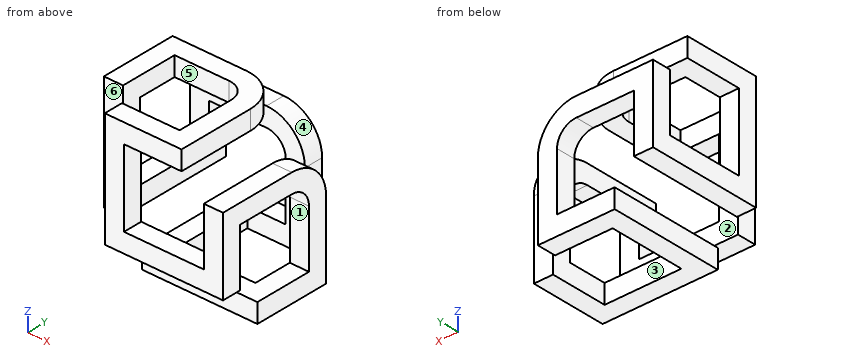
```python
from build123d import *

# Parameters (mm, degrees)
SKETCH_1_W      = 10
SKETCH_1_H      = 10
EXTRUDE_1_DEPTH = 10
EXTRUDE_2_DEPTH = 10
EXTRUDE_3_DEPTH = 10
EXTRUDE_4_DEPTH = 10
EXTRUDE_5_DEPTH = 10
EXTRUDE_6_DEPTH = 10
FILLET_3_R      = 20
FILLET_4_R      = 10
FILLET_5_R      = 20
FILLET_6_R      = 20
FILLET_7_R      = 10
FILLET_8_R      = 10


with BuildPart() as part:
    # 草图1 → 凸台-拉伸1 (new body)
    with BuildSketch(Plane.XY):
        Polygon((0, 60), (0, 30), (10, 30), (10, 50), (48.396471527, 50), (48.396471527, 10), (28.396471527, 10), (28.396471527, 0), (58.396471527, 0), (58.396471527, 60), align=None)
        with Locations((5, 25)):
            Rectangle(SKETCH_1_W, SKETCH_1_H)
        with Locations((23.396471527, 5)):
            Rectangle(SKETCH_1_W, SKETCH_1_H)
    extrude(amount=-EXTRUDE_1_DEPTH)

    # 草图2 → 凸台-拉伸2 (add)
    with BuildSketch(Plane.ZY):
        Polygon((0, 20), (-60, 20), (-60, 80), (-20, 80), (-20, 70), (-50, 70), (-50, 30), (-10, 30), (-10, 60), (0, 60), align=None)
    extrude(amount=-EXTRUDE_2_DEPTH)

    # 草图3 → 凸台-拉伸3 (add)
    with BuildSketch(Plane(origin=(0, 80, 0), x_dir=(1, 0, 0), z_dir=(0, 1, 0))):
        Polygon((0, 60), (0, 20), (60, 20), (60, 80), (20, 80), (20, 70), (50, 70), (50, 30), (10, 30), (10, 60), align=None)
    extrude(amount=-EXTRUDE_3_DEPTH)

    # 草图4 → 凸台-拉伸4 (add)
    with BuildSketch(Plane(origin=(0, 0, -80), x_dir=(-1, 0, 0), z_dir=(0, 0, -1))):
        Polygon((-60, 80), (-20, 80), (-20, 20), (-80, 20), (-80, 60), (-70, 60), (-70, 30), (-30, 30), (-30, 70), (-60, 70), align=None)
    extrude(amount=-EXTRUDE_4_DEPTH)

    # 草图5 → 凸台-拉伸5 (add)
    with BuildSketch(Plane(origin=(80, 0, 0), x_dir=(0, 0, -1), z_dir=(1, 0, 0))):
        Polygon((80, 60), (20, 60), (20, 0), (60, 0), (60, 10), (30, 10), (30, 50), (70, 50), (70, 20), (80, 20), align=None)
    extrude(amount=-EXTRUDE_5_DEPTH)

    # 草图6 → 凸台-拉伸6 (add)
    with BuildSketch(Plane.XZ):
        Polygon((18.396471527, -10), (18.396471527, -60), (70, -60), (70, -50), (28.396471527, -50), (28.396471527, -10), align=None)
    extrude(amount=-EXTRUDE_6_DEPTH)

    # 圆角3
    fillet_3_edges = [part.edges().sort_by_distance(p)[0] for p in [
        (60, 75, -20),
    ]]
    fillet(fillet_3_edges, radius=FILLET_3_R)

    # 圆角4
    fillet_4_edges = [part.edges().sort_by_distance(p)[0] for p in [
        (50, 75, -30),
    ]]
    fillet(fillet_4_edges, radius=FILLET_4_R)

    # 圆角5
    fillet_5_edges = [part.edges().sort_by_distance(p)[0] for p in [
        (75, 60, -20),
    ]]
    fillet(fillet_5_edges, radius=FILLET_5_R)

    # 圆角6
    fillet_6_edges = [part.edges().sort_by_distance(p)[0] for p in [
        (58.396471527, 60, -5),
    ]]
    fillet(fillet_6_edges, radius=FILLET_6_R)

    # 圆角7
    fillet_7_edges = [part.edges().sort_by_distance(p)[0] for p in [
        (48.396471527, 50, -5),
    ]]
    fillet(fillet_7_edges, radius=FILLET_7_R)

    # 圆角8
    fillet_8_edges = [part.edges().sort_by_distance(p)[0] for p in [
        (75, 50, -30),
    ]]
    fillet(fillet_8_edges, radius=FILLET_8_R)


solid = part.part
```
Geometry: final body of the model. Coordinates: model frame, mm. Face numbers are marked on the shaded views. A direction names the side the tool comes from. Give positions to 0.01 mm unless a question says otherwise; leave off trailing zeros. Loops run counter-clockwise (first coordinate to the right, second up) from the corner with the lowest first, then second, coordinate; pieces in that order, holes last. Notation, with made-up numbers: (10, -5) - (33, -5) arc R10 ccw to (33, 8) - close; hole circle Ø3 at (-4, 9). An arc over 180 degrees is marked (long way). Answer as CSV lines item,"result". Start each with the question number.
(1) Mould query, pull axis X, two halves, no side actions, for the marked faces 4, 5 and 6. Classes: +X half, -X half, draft (parallel to the pull), parting line (faces both ways), or undercut.
(2) Section query C-C (x = 21.5). Output: boundary loops of the cut face in (y, z), and give its area (3 significant figures).
(3) Section query D-D (z = -46). Output: boundary loops of the cut face in (x, y), and give its area (3 significant figures).
(4) Section query A-A (y = 68). Output: boundary loops of the cut face in (x, z).
(5) Ray query, line 1 along Z through (x, y) = (9, 45); line 2 along X through (y, z) = (37.5, -7.5); line 3 along X through (y, z) = (72.5, -59). Return the intervals inside material, ascending. Write a range as [from, to].
(6) Pin query (flat end, axial travel): P1, Ø5, axis at x = 49, z = -46.5, coming from the -Y side; P2, Ø12, axis at x = 26.5, y = 27.5, coming from the +Z side; P3, Ø11, axis at y = 15.5, z = -7, coming from the +X side; P4, Ø2, axis at y = 57.5, z = -11.5, coming from the -X side. Return the tip coordinate at first contact, or that it passes through.
(7) Section query B-B (z = -28). Output: boundary loops of the cut face in (x, y).
(8) Reachability of the marked faces 1, 2 and 3 from +Z, -Z, +X, -X, +Y, -Y: full face, straight path, thin tool, end or side. Return the list, or none.
Worked answers:
1,face 4,"+X half"
1,face 5,"undercut"
1,face 6,"draft"
2,outline,"(0, -60) - (10, -60) - (10, 0) - (0, 0) - close; (20, -80) - (80, -80) - (80, -70) - (20, -70) - close; (50, -10) - (60, -10) - (60, 0) - (50, 0) - close; (70, -30) - (80, -30) - (80, -20) - (70, -20) - close"
2,area,"1,400 mm^2"
3,outline,"(0, 20) - (10, 20) - (10, 30) - (0, 30) - close; (0, 70) - (10, 70) - (10, 80) - (0, 80) - close; (18.4, 0) - (28.4, 0) - (28.4, 10) - (18.4, 10) - close; (50, 70) - (60, 70) - (60, 80) - (50, 80) - close; (70, 0) - (80, 0) - (80, 10) - (70, 10) - close; (70, 50) - (80, 50) - (80, 60) - (70, 60) - close"
3,area,"600 mm^2"
4,outline,"(0, -60) - (10, -60) - (10, -50) - (0, -50) - close; (20, -80) - (30, -80) - (30, -70) - (20, -70) - close"
5,line 1,"z = [-60, -50], [-10, 0]"
5,line 2,"x = [0, 10], [48.4, 58.4]"
5,line 3,"x = [0, 10], [50, 60]"
6,P1,"stops at y = 70"
6,P2,"stops at z = -70"
6,P3,"stops at x = 58.4"
6,P4,"passes through"
7,outline,"(0, 20) - (10, 20) - (10, 30) - (0, 30) - close; (0, 70) - (56, 70) - (56, 80) - (0, 80) - close; (18.4, 0) - (28.4, 0) - (28.4, 10) - (18.4, 10) - close; (70, 0) - (80, 0) - (80, 56) - (70, 56) - close"
8,face 1,"+X"
8,face 2,"-Z, -X"
8,face 3,"-Z"
